Source: CAD feature listing. Evaluate the final solid. Frame: model axes, mm. Face numbers are marked on the shaded views. A direction names the side the tool comes from. Give positions to 0.01 mm unless a question says otherwise; leave off trailing zeros. Write each loop counter-clockwise with the first axis right and the second up, starting at its lowest first coordinate (ties: lowest second). Pieces come first, ordered by that corner, then holes. Notation, with made-up numbers: (83.5, 39.5) - (112.5, 39.5) arc R17 ccw to (112.5, 60.5) - close; hole circle Ø3 at (28.25, 0.25). An arc over 180 degrees is marked (long way). Answer as a JSON object with one key per item and string values. Group by question number.
Autodesk Inventor part; units mm, degrees
ref_plane "YZ Plane" through (0, 0, 0) normal (1, 0, 0) x (0, 1, 0)
ref_plane "XZ Plane" through (0, 0, 0) normal (0, 1, 0) x (-1, 0, 0)
ref_plane "XY Plane" through (0, 0, 0) normal (0, 0, 1) x (1, 0, 0)
sketch "Sketch1" plane through (0, 0, 0) normal (0, 1, 0) x (-1, 0, 0)
  line L0 (0, 0) -> (1524, 0)
  line L1 (1524, 0) -> (1524, -1524)
  line L2 (1524, -1524) -> (0, -1524)
  line L3 (0, -1524) -> (0, 0)
  line L4 (1517.65, -1517.65) -> (6.35, -1517.65)
  line L5 (6.35, -1517.65) -> (6.35, -6.35)
  line L6 (6.35, -6.35) -> (1517.65, -6.35)
  line L7 (1517.65, -6.35) -> (1517.65, -1517.65)
  dimension "d0" = 1524
  dimension "d1" = 1524
  dimension "d4" = 6.35
  dimension "d5" = 6.35
  dimension "d6" = 6.35
  dimension "d7" = 6.35
extrude "Extrusion2" add sketch "Sketch1" along normal blind 1981.2
sketch "Sketch2" plane through (0, 1981.2, 0) normal (0, 1, 0) x (1, 0, 0)
  line L0 (0, 1524) -> (-1524, 1524)
  line L1 (0, 0) -> (-1524, 0)
  line L2 (-1524, 0) -> (-1524, 1524)
  line L3 (-1524, 1524) -> (0, 1524)
  line L4 (0, 1524) -> (0, 0)
extrude "Extrusion3" add sketch "Sketch2" along normal blind 6.35
sketch "Sketch3" plane through (0, 0, 0) normal (0, -1, 0) x (1, 0, 0)
  line L0 (0, 0) -> (0, -1524)
  line L1 (0, -1524) -> (-1524, -1524)
  line L2 (0, 0) -> (-1524, 0)
  line L3 (-1524, 0) -> (-1524, -1524)
  line L4 (-1524, -1524) -> (0, -1524)
  line L5 (0, -1524) -> (0, 0)
extrude "Extrusion4" add sketch "Sketch3" along normal blind 6.35
sketch "Sketch5" plane through (-1524, 1987.55, -1524) normal (-1, 0, 0) x (0, 0, 1)
  line L0 (1371.6, -234.95) -> (152.4, -234.95)
  line L1 (152.4, -234.95) -> (152.4, -1758.95)
  line L2 (152.4, -1758.95) -> (1371.6, -1758.95)
  line L3 (1371.6, -1758.95) -> (1371.6, -234.95)
  line L4 (1524, -1993.9) -> (1524, 0)
  line L5 (1524, -1993.9) -> (0, -1993.9)
  point P0 (1524, -1987.55)
  dimension "d21" = 1219.2
  dimension "d22" = 1524
  dimension "d23" = 152.4
  dimension "d24" = 234.95
extrude "Extrusion6" cut sketch "Sketch5" against normal through all
properties part number "ASTRA_Body" material "Aluminum 6061"
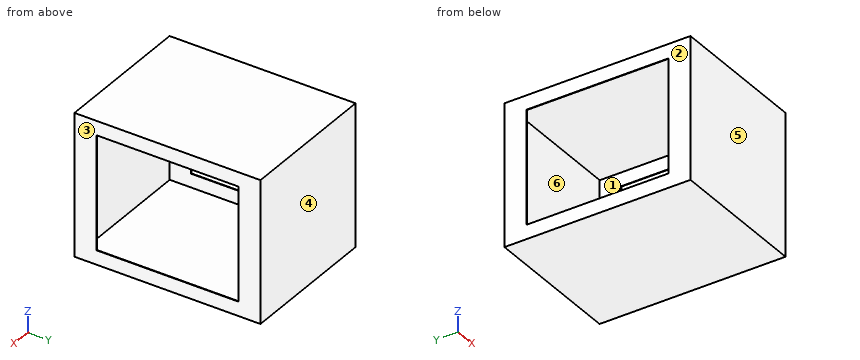
Q1. Reachability of the marked faces 1 and 2 from +Z, -Z, +X, -X, +Y, -Y: full face, straight path, thin tool, end or side. Return the list, or none.
Q2. First-contact query: pin 1 Ø1.5 at (x, y) = (-493.5, 1554.5) entering from +Z. Flat tip, straight axial feed; report the tip coordinate or a pass-through.
Q3. Draft query along Y for the marked faces 3, 4, 5 and 6. Return one class per face: released by +Y, released by -Y, zero draft, split by the parting line, or undercut.
Q4. Section B-B on z = -1239. Return the cut outline in (x, y).
Q5. Section C-C on x = -1015.5. Return the cut outline in (y, z), then the cut area to 3 significant figures.
Q6. Section A-A on y = 1618. Return the cut outline in (x, z).
Q7. Ray query, probe 1 along Z at (x, y) = (-265.5, 379); probe 2 along Y at (x, z) = (-266.5, -681). Return the intervals inside material, ascending. Write a range as [from, to].
Taken from the geometry:
{
 "1": {"face 1": "none", "face 2": "+Z, -Z, -X, +Y, -Y"},
 "2": {"pin 1": "stops at z = 0"},
 "3": {"face 3": "zero draft", "face 4": "released by +Y", "face 5": "released by -Y", "face 6": "undercut"},
 "4": {"outline": "(-1524, -6.35) - (0, -6.35) - (0, 228.6) - (-6.35, 228.6) - (-6.35, 0) - (-1517.65, 0) - (-1517.65, 228.6) - (-1524, 228.6) - close; (-1524, 1752.6) - (-1517.65, 1752.6) - (-1517.65, 1981.2) - (-6.35, 1981.2) - (-6.35, 1752.6) - (0, 1752.6) - (0, 1987.55) - (-1524, 1987.55) - close"},
 "5": {"outline": "(-6.35, -1524) - (1987.55, -1524) - (1987.55, 0) - (-6.35, 0) - close; hole (0, -1517.65) - (1981.2, -1517.65) - (1981.2, -6.35) - (0, -6.35) - close", "area": "44,500 mm²"},
 "6": {"outline": "(-1524, -1524) - (0, -1524) - (0, -1371.6) - (-6.35, -1371.6) - (-6.35, -1517.65) - (-1517.65, -1517.65) - (-1517.65, -1371.6) - (-1524, -1371.6) - close; (-1524, -152.4) - (-1517.65, -152.4) - (-1517.65, -6.35) - (-6.35, -6.35) - (-6.35, -152.4) - (0, -152.4) - (0, 0) - (-1524, 0) - close"},
 "7": {"probe 1": "z = [-1524, -1517.65], [-6.35, 0]", "probe 2": "y = [-6.35, 0], [1981.2, 1987.55]"}
}
